Autodesk Inventor part; units mm, degrees
ref_plane "cut1_XY" through (12.7, 6.2865, 0) normal (1, 0, 0) x (0, 0, -1)
ref_plane "cut1_YZ" through (12.7, 6.2865, 0) normal (0, 0, -1) x (0, 1, 0)
ref_plane "cut1_ZX" through (12.7, 6.2865, 0) normal (0, 1, 0) x (1, 0, 0)
sketch "Sketch_1" plane through (0, 0, 0) normal (0, 0, 1) x (1, 0, 0)
  line L0 (12.7, 0) -> (0, 0)
  line L1 (0, 0) -> (0, 6.5088)
  line L2 (0, 6.5088) -> (0.762, 7.2708)
  line L3 (0.762, 7.2708) -> (2.7178, 7.2708)
  line L4 (2.7178, 7.2708) -> (3.3528, 6.6357)
  line L5 (3.3528, 6.6357) -> (3.9878, 6.6357)
  line L6 (3.9878, 6.6357) -> (3.9878, 7.7407)
  line L7 (3.9878, 7.7407) -> (11.938, 7.7407)
  line L8 (11.938, 7.7407) -> (12.7, 6.9787)
  line L9 (12.7, 6.9787) -> (12.7, 0)
  line L10 (12.7, 0) -> (0, 0)
revolve "Revolution1" add sketch "Sketch_1" angle 360 about axis through (12.7, 0, 0) along (1, 0, 0)
sketch "Sketch2" plane through (12.7, 0, 0) normal (1, 0, 0) x (0, 0, -1)
  point P0 (0, 0)
hole "Drilling 1" at (12.7, 0, 0) direction (-1, 0, 0) diameter 7.9248 depth 0.381
sketch "Sketch3" plane through (12.319, 0, 0) normal (1, 0, 0) x (0, 0, -1)
  point P0 (0, 0)
hole "Drilling 2" at (12.319, 0, 0) direction (-1, 0, 0) diameter 3.9624 depth 12.319 countersink diameter 4.826 countersink angle 90
sketch "Sketch_5" plane through (12.7, 0, 0) normal (1, 0, 0) x (0, 0, -1)
  line L0 (-30.9626, 15.4813) -> (-30.9626, -15.4813)
  line L1 (-30.9626, -15.4813) -> (30.9626, -15.4813)
  line L2 (30.9626, -15.4813) -> (30.9626, 15.4813)
  line L3 (30.9626, 15.4813) -> (-30.9626, 15.4813)
  line L4 (-15.4813, 6.2865) -> (-15.4813, -6.2865)
  line L5 (-15.4813, -6.2865) -> (15.4813, -6.2865)
  line L6 (15.4813, -6.2865) -> (15.4813, 6.2865)
  line L7 (15.4813, 6.2865) -> (-15.4813, 6.2865)
extrude "Extrusion1" cut sketch "Sketch_5" against normal blind 4.826
sketch "Sketch_24" plane through (0, 0, 0) normal (0, 0, 1) x (1, 0, 0)
  line L0 (3.9878, 0) -> (3.3528, 0)
  line L1 (3.2301, 7.6565) -> (3.8708, 7.0158)
  arc A0 (3.8708, 6.8362) -> (3.8708, 7.0158) centre (3.781, 6.926) ccw
  line L2 (3.8708, 6.8362) -> (3.6703, 6.6357)
  line L3 (3.6703, 6.6357) -> (3.3528, 6.6357)
  line L4 (3.3528, 6.6357) -> (3.3528, 6.3818)
  line L5 (3.3528, 6.3818) -> (3.9878, 6.3818)
  line L6 (3.9878, 6.3818) -> (3.9878, 7.1861)
  line L7 (3.9878, 7.1861) -> (3.4333, 7.7407)
  line L8 (3.4333, 7.7407) -> (3.2301, 7.7407)
  line L9 (3.2301, 7.7407) -> (3.2301, 7.6565)
revolve "Revolution2" add sketch "Sketch_24" angle 360 about axis through (3.9878, 0, 0) along (1, 0, 0)
ref_plane "cut1_XY" through (12.7, 6.2865, 0) normal (1, 0, 0) x (0, 0, -1)
ref_plane "cut1_YZ" through (12.7, 6.2865, 0) normal (0, 0, -1) x (0, 1, 0)
ref_plane "cut1_ZX" through (12.7, 6.2865, 0) normal (0, 1, 0) x (1, 0, 0)
ref_plane "cut2_XY" through (12.7, -6.2865, 0) normal (1, 0, 0) x (0, 0, -1)
ref_plane "cut2_YZ" through (12.7, -6.2865, 0) normal (0, 0, -1) x (0, 1, 0)
ref_plane "cut2_ZX" through (12.7, -6.2865, 0) normal (0, 1, 0) x (1, 0, 0)
ref_plane "to_tube_XY" through (3.3528, 0, 0) normal (1, 0, 0) x (0, 0, -1)
ref_plane "to_tube_YZ" through (3.3528, 0, 0) normal (0, 0, -1) x (0, 1, 0)
ref_plane "to_tube_ZX" through (3.3528, 0, 0) normal (0, 1, 0) x (1, 0, 0)
ref_plane "lovra_XY" through (12.7, 0, 0) normal (1, 0, 0) x (0, 1, 0)
ref_plane "lovra_YZ" through (12.7, 0, 0) normal (0, 1, 0) x (0, 0, 1)
ref_plane "lovra_ZX" through (12.7, 0, 0) normal (0, 0, 1) x (1, 0, 0)
ref_plane "to_nut_XY" through (0, 0, 0) normal (1, 0, 0) x (0, 0, -1)
ref_plane "to_nut_YZ" through (0, 0, 0) normal (0, 0, -1) x (0, 1, 0)
ref_plane "to_nut_ZX" through (0, 0, 0) normal (0, 1, 0) x (1, 0, 0)
ref_plane "lovra1_XY" through (7.874, 0, 0) normal (1, 0, 0) x (0, 0, -1)
ref_plane "lovra1_YZ" through (7.874, 0, 0) normal (0, 0, -1) x (0, 1, 0)
ref_plane "lovra1_ZX" through (7.874, 0, 0) normal (0, 1, 0) x (1, 0, 0)
ref_plane "lovra2_XY" through (7.874, 6.2865, 0) normal (1, 0, 0) x (0, 0, -1)
ref_plane "lovra2_YZ" through (7.874, 6.2865, 0) normal (0, 0, -1) x (0, 1, 0)
ref_plane "lovra2_ZX" through (7.874, 6.2865, 0) normal (0, 1, 0) x (1, 0, 0)
ref_plane "lovra3_XY" through (7.874, -6.2865, 0) normal (1, 0, 0) x (0, 0, -1)
ref_plane "lovra3_YZ" through (7.874, -6.2865, 0) normal (0, 0, -1) x (0, 1, 0)
ref_plane "lovra3_ZX" through (7.874, -6.2865, 0) normal (0, 1, 0) x (1, 0, 0)
ref_plane "olen_XY" through (12.7, 0, 0) normal (1, 0, 0) x (0, 0, -1)
ref_plane "olen_YZ" through (12.7, 0, 0) normal (0, 0, -1) x (0, 1, 0)
ref_plane "olen_ZX" through (12.7, 0, 0) normal (0, 1, 0) x (1, 0, 0)
ref_plane "cutf1_XY" through (12.7, 7.7407, 0) normal (0, 0, 1) x (1, 0, 0)
ref_plane "cutf1_YZ" through (12.7, 7.7407, 0) normal (1, 0, 0) x (0, 1, 0)
ref_plane "cutf1_ZX" through (12.7, 7.7407, 0) normal (0, 1, 0) x (0, 0, 1)
ref_plane "cutf2_XY" through (7.874, 7.7407, 0) normal (0, 0, 1) x (1, 0, 0)
ref_plane "cutf2_YZ" through (7.874, 7.7407, 0) normal (1, 0, 0) x (0, 1, 0)
ref_plane "cutf2_ZX" through (7.874, 7.7407, 0) normal (0, 1, 0) x (0, 0, 1)
ref_plane "lovra21_XY" through (0, 0, 5.2705) normal (1, 0, 0) x (0, 0, -1)
ref_plane "lovra21_YZ" through (0, 0, 5.2705) normal (0, 0, -1) x (0, 1, 0)
ref_plane "lovra21_ZX" through (0, 0, 5.2705) normal (0, 1, 0) x (1, 0, 0)
ref_plane "lovra22_XY" through (0, 0, -5.2705) normal (1, 0, 0) x (0, 0, -1)
ref_plane "lovra22_YZ" through (0, 0, -5.2705) normal (0, 0, -1) x (0, 1, 0)
ref_plane "lovra22_ZX" through (0, 0, -5.2705) normal (0, 1, 0) x (1, 0, 0)
ref_plane "to_pin_XY" through (19.8374, 0, 0) normal (0, 0, 1) x (1, 0, 0)
ref_plane "to_pin_YZ" through (19.8374, 0, 0) normal (1, 0, 0) x (0, 1, 0)
ref_plane "to_pin_ZX" through (19.8374, 0, 0) normal (0, 1, 0) x (0, 0, 1)
ref_plane "mbr_XY" through (13.5128, 0, 0) normal (1, 0, 0) x (0, 0, -1)
ref_plane "mbr_YZ" through (13.5128, 0, 0) normal (0, 0, -1) x (0, 1, 0)
ref_plane "mbr_ZX" through (13.5128, 0, 0) normal (0, 1, 0) x (1, 0, 0)
ref_plane "to_nut1_XY" through (15.0876, 0, 0) normal (1, 0, 0) x (0, 0, -1)
ref_plane "to_nut1_YZ" through (15.0876, 0, 0) normal (0, 0, -1) x (0, 1, 0)
ref_plane "to_nut1_ZX" through (15.0876, 0, 0) normal (0, 1, 0) x (1, 0, 0)
properties part number "02R00_NR_rear_head"
The model under review builds one solid part; all positions refer to its coordinate system, in mm. A direction names the side the tool comes from. Coordinates: 2 decimals unless noted, no trailing zeros. Write each loop counter-clockwise with the first axis right and the second up, starting at its lowest first coordinate (ties: lowest second). Pieces come first, ordered by that corner, then holes. Notation, with made-up numbers: (-10, 33) - (30, 33) arc R20 ccw to (30, 39) - close; hole circle Ø9 at (52, 60). An arc over 180 degrees is marked (long way). Answer in a Markdown table with one row per item. Add a question column.
Q1. Clearance check with flat-ended pins moving along their axes: pin 1 (2.5 mm diameter, centred on x = 9.5, z = 1.5, fed in from +Y); pin 2 (4 mm diameter, centred on y = 0, z = -1.5, fed in from -X); pin 3 (2 mm diameter, centred on x = 9, y = -1.5, fed in from -Z); pin 4 (2.5 mm diameter, centred on x = 10, z = -0.5, fed in from -Y). State where each tip first meets the part, or that it passes through.
Q2. Consider section A-A on x = 10.25. Give the boundary of the cut face in (y, z), then the cut area to 3 significant figures.
Q3. Draft analysis for pull direction X (two halves, no side actions). For faces 1 (the face through (10, 6.286, 0)), 2 (the face through (12.57, 0.11, -7.11)), 3 (the face through (3.51, -0.86, 6.58)), state which applies: +X half, -X half, draft (parallel to the pull), parting line (faces both ways), or undercut.
Q4. For faces 4 (the face through (12.7, -3, 3)), 5 (the face through (1.754, -5.77, -4.424)), 6 (the face through (10, -6.286, 0)), list the 3-axis set-ups (+Z, -Z, +X, -X, +Y, -Y) from which the entire face can be reached by the end or side of a thin tool; tool diameter is ignored.
Q5. Consider section B-B on x = 5. Give the boundary of the cut face in (y, z), then the cut area to 3 significant figures.
Q6. To check wall thickness, follow line 1 along Z through (x, y) = (8, 0); line 2 along Y through (x, z) = (12.5, 0); line 3 along Y through (x, z) = (9.5, 0). State the ranges of each line that lie inside material, in increasing order. Write a range as from..to.
Answers below:
| question | item | result |
|---|---|---|
| 1 | pin 1 | y = 6.29 |
| 1 | pin 2 | x = 0 |
| 1 | pin 3 | z = -7.72 |
| 1 | pin 4 | y = -6.29 |
| 2 | outline | (-6.29, -4.52) arc R7.74 ccw to (6.29, -4.52) - (6.29, 4.52) arc R7.74 ccw to (-6.29, 4.52) - close; hole circle Ø3.96 at (0, 0) |
| 2 | area | 158 mm² |
| 3 | face 1 | draft |
| 3 | face 2 | +X half |
| 3 | face 3 | undercut |
| 4 | face 4 | +Z, -Z, +X, +Y, -Y |
| 4 | face 5 | -X |
| 4 | face 6 | +Z, -Z, +X, -Y |
| 5 | outline | circle Ø15.48 at (0, 0); hole circle Ø3.96 at (0, 0) |
| 5 | area | 176 mm² |
| 6 | line 1 | -7.74..-1.98, 1.98..7.74 |
| 6 | line 2 | -6.29..-3.96, 3.96..6.29 |
| 6 | line 3 | -6.29..-1.98, 1.98..6.29 |
